The figure shows three views and two pictorial views of one solid part (mm, origin at its lowest corner). Answer the questions. A direction names the side the tool comes from. Coordinates: 2 decimals unless noted, no trailing zeros. Loops run counter-clockwise (first coordinate to the right, second up) from the corner with the lowest first, then second, coordinate; pieces in that order, holes last. Notation, with made-up numbers: (85, 60.25) - (120, 60.25) arc R21 ccw to (120, 79.25) - close; hole circle Ø8 at (84, -24.5). An arc over 180 degrees is marked (long way). Write each question's results on one line, items separated by ' | '. Start each with the question number.
Item 1: Section A-A, the plane x = 31.75 is taken. Write down the section's boundary in (y, z) (3 decimals), plus the area to 3 significant figures.
Item 2: Section C-C, the plane z = 30.5 is taken. Write down the section's boundary in (x, y), plus the area to 3 significant figures.
Item 3: Each of these flat-tipped pins is pushed along its axis until it touches: pin 1 Ø1 at (x, y) = (42.5, 89) entering from +Z; pin 2 Ø5 at (y, z) = (199, 29) entering from -X; pin 3 Ø14.5 at (x, y) = (31.75, 234.95) entering from -Z; pin 4 Ø8 at (x, z) = (47.5, 48.5) entering from -Y. Where does it stop, or does it pass through?
Item 4: Section D-D, the plane y = 19.05 is taken. Write down the section's boundary in (x, z) (3 decimals), plus the area to 3 significant figures.
Item 5: A tool of negligible diameter and unlimited length cuts with its end or side. For the marked faces 1 and 2, from which of +Z, -Z, +X, -X, +Y, -Y can it reach the whole face along a straight path? Write none if from no direction.
Item 6: Consider probe 1 along Y at (x, z) = (31, 72); probe 2 along Z at (x, y) = (10.5, 232.5); probe 3 along Z at (x, y) = (15.5, 50.5). Determine where each line is inside the solid, lowest interval first. Write a range as [from, to].
Item 7: For a pull along Z with two mould halves and no side action, classify the marked faces 3, 4 and 5 as +Z half, -Z half, draft (parallel to the pull), parting line (faces both ways), or undercut.
Item 8: Section B-B, the plane y = 234.95 is taken. Write down the section's boundary in (x, z).
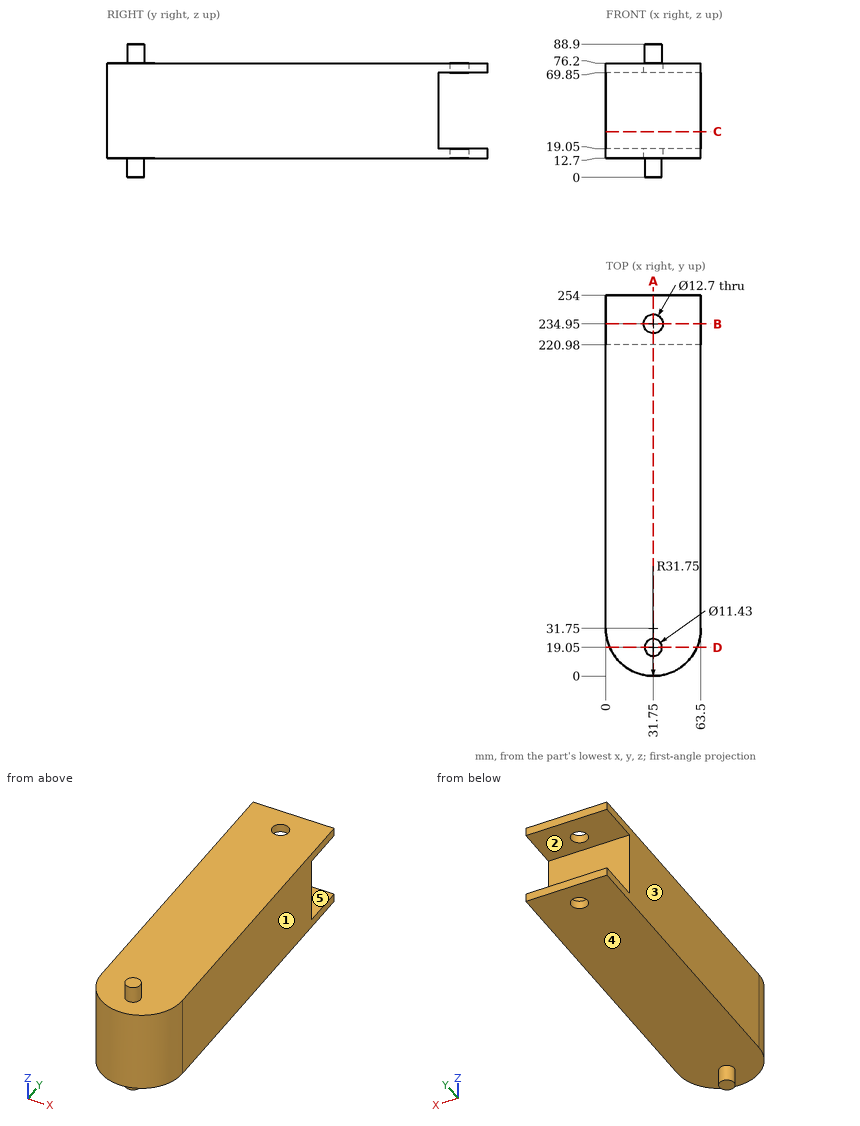
Answer key:
1) outline: (0, 12.7) - (13.335, 12.7) - (13.335, 0) - (24.765, 0) - (24.765, 12.7) - (228.6, 12.7) - (228.6, 19.05) - (220.98, 19.05) - (220.98, 69.85) - (228.6, 69.85) - (228.6, 76.2) - (24.765, 76.2) - (24.765, 88.9) - (13.335, 88.9) - (13.335, 76.2) - (0, 76.2) - close; (241.3, 12.7) - (254, 12.7) - (254, 19.05) - (241.3, 19.05) - close; (241.3, 69.85) - (254, 69.85) - (254, 76.2) - (241.3, 76.2) - close | area: 14,600 mm^2
2) outline: (0, 31.75) arc R31.75 ccw to (63.5, 31.75) - (63.5, 220.98) - (0, 220.98) - close | area: 13,600 mm^2
3) pin 1: stops at z = 76.2 | pin 2: stops at x = 0 | pin 3: stops at z = 12.7 | pin 4: stops at y = 2.25
4) outline: (2.651, 12.7) - (26.035, 12.7) - (26.035, 0) - (37.465, 0) - (37.465, 12.7) - (60.849, 12.7) - (60.849, 76.2) - (37.465, 76.2) - (37.465, 88.9) - (26.035, 88.9) - (26.035, 76.2) - (2.651, 76.2) - close | area: 3,990 mm^2
5) face 1: +Z, -Z, +X, +Y, -Y | face 2: +X, -X, +Y
6) probe 1: y = [0.01, 228.64], [241.26, 254] | probe 2: z = [12.7, 19.05], [69.85, 76.2] | probe 3: z = [12.7, 76.2]
7) face 3: draft | face 4: -Z half | face 5: undercut
8) outline: (0, 12.7) - (25.4, 12.7) - (25.4, 19.05) - (0, 19.05) - close; (0, 69.85) - (25.4, 69.85) - (25.4, 76.2) - (0, 76.2) - close; (38.1, 12.7) - (63.5, 12.7) - (63.5, 19.05) - (38.1, 19.05) - close; (38.1, 69.85) - (63.5, 69.85) - (63.5, 76.2) - (38.1, 76.2) - close
